from build123d import *

# Parameters (mm, degrees)
SKETCH1_W           = 15.9512
SKETCH1_H           = 13.3096
BOSS_EXTRUDE1_DEPTH = 1.6764
SKETCH2_W           = 2.794
SKETCH2_H           = 1.27
BOSS_EXTRUDE2_DEPTH = 1.016
SKETCH3_R           = 0.9525
CUT_EXTRUDE1_DEPTH  = 2.6764


with BuildPart() as part:
    # Sketch1 → Boss-Extrude1 (new body)
    with BuildSketch(Plane(origin=(0, 0, 0), x_dir=(1, 0, 0), z_dir=(0, 1, 0))):
        with Locations((7.9756, 6.6548)):
            Rectangle(SKETCH1_W, SKETCH1_H)
    extrude(amount=BOSS_EXTRUDE1_DEPTH)

    # Sketch2 → Boss-Extrude2 (add)
    with BuildSketch(Plane(origin=(0, 1.6764, 0), x_dir=(1, 0, 0), z_dir=(0, 1, 0))):
        with Locations((2.413, 6.6548)):
            Rectangle(SKETCH2_W, SKETCH2_H)
        with Locations((6.223, 6.6548)):
            Rectangle(SKETCH2_W, SKETCH2_H)
        with Locations((9.7282, 6.6548)):
            Rectangle(SKETCH2_W, SKETCH2_H)
        with Locations((13.5382, 6.6548)):
            Rectangle(SKETCH2_W, SKETCH2_H)
    extrude(amount=BOSS_EXTRUDE2_DEPTH)

    # Sketch3 → Cut-Extrude1 (cut, through all)
    with BuildSketch(Plane(origin=(0, 1.6764, 0), x_dir=(1, 0, 0), z_dir=(0, 1, 0))):
        with Locations((1.329266667, 12.0396)):
            Circle(SKETCH3_R)
        with Locations((3.987808467, 12.0396)):
            Circle(SKETCH3_R)
        with Locations((6.646350267, 12.0396)):
            Circle(SKETCH3_R)
        with Locations((9.304892067, 12.0396)):
            Circle(SKETCH3_R)
        with Locations((11.963433867, 12.0396)):
            Circle(SKETCH3_R)
        with Locations((14.621975667, 12.0396)):
            Circle(SKETCH3_R)
        with Locations((14.621975667, 1.27)):
            Circle(SKETCH3_R)
        with Locations((11.963433867, 1.27)):
            Circle(SKETCH3_R)
        with Locations((9.304892067, 1.27)):
            Circle(SKETCH3_R)
        with Locations((6.646350267, 1.27)):
            Circle(SKETCH3_R)
        with Locations((3.987808467, 1.27)):
            Circle(SKETCH3_R)
        with Locations((1.329266667, 1.27)):
            Circle(SKETCH3_R)
    extrude(amount=-CUT_EXTRUDE1_DEPTH, mode=Mode.SUBTRACT)


solid = part.part
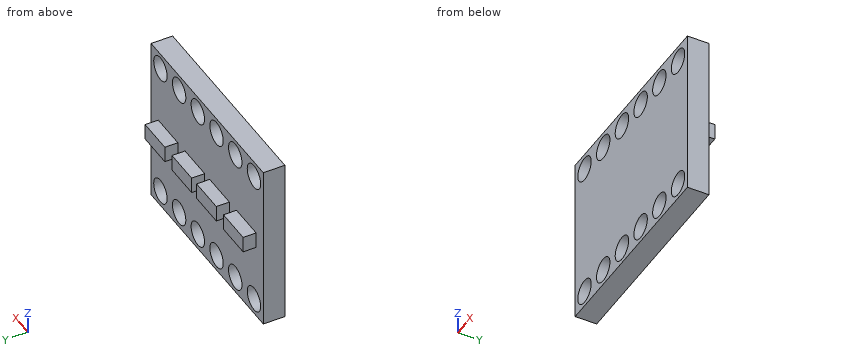
Work out the finished part from the listing and answer in its coordinate system (mm). Give positions to 0.01 mm unless a question says otherwise; leave off trailing zeros. Loops run counter-clockwise (first coordinate to the right, second up) from the corner with the lowest first, then second, coordinate; pieces in that order, holes last. Notation, with made-up numbers: (77.25, 26.25) -> (94.25, 26.25) arc R11 cw to (94.25, 39.25) -> close; hole circle Ø3 at (30, -5). An arc over 180 degrees is marked (long way). Use a Markdown table: item, result. Add a question column.
1) Consider line 1 along Z through (x, y) = (12.5, 1.2); line 2 along Z through (x, y) = (4.25, 1.2); line 3 along Y through (x, z) = (11.75, -4). Determine where each line is inside the solid, lowest interval first.
2) The part is cut by section B-B, the plane z = -1.27. Determine the outline of the cut face in (x, y).
3) The part is cut by section A-A, the plane y = 2.15. Determine the outline of the cut face in (x, z).
4) Each of these flat-tipped pins is pushed along its axis until it touches: P1, Ø3, axis at x = 3.99, z = -1.27, coming from the +Y side; P2, Ø0.8, axis at y = 2.5, z = -6.5, coming from the +X side; P3, Ø0.5, axis at x = 6.5, y = 2, coming from the +Z side. Where does it stop, or does it pass through?
5) The part is cut by section C-C, the plane x = 4. Determine the outline of the cut face in (y, z), plus the area to 3 significant figures.
6) The part is cut by section D-D, the plane y = 0.4. Count the separate pieces of the cut face and the enclosed holes in it, plus the area to 3 significant figures.
Reported:
| question | item | result |
|---|---|---|
| 1 | line 1 | z = -13.31 to -12.83, -11.25 to -2.06, -0.48 to 0 |
| 1 | line 2 | z = -13.31 to -12.96, -11.12 to -2.19, -0.35 to 0 |
| 1 | line 3 | y = 0 to 1.68 |
| 2 | outline | (0, 0) -> (0.38, 0) -> (0.38, 1.68) -> (0, 1.68) -> close; (2.28, 0) -> (3.04, 0) -> (3.04, 1.68) -> (2.28, 1.68) -> close; (4.94, 0) -> (5.69, 0) -> (5.69, 1.68) -> (4.94, 1.68) -> close; (7.6, 0) -> (8.35, 0) -> (8.35, 1.68) -> (7.6, 1.68) -> close; (10.26, 0) -> (11.01, 0) -> (11.01, 1.68) -> (10.26, 1.68) -> close; (12.92, 0) -> (13.67, 0) -> (13.67, 1.68) -> (12.92, 1.68) -> close; (15.57, 0) -> (15.95, 0) -> (15.95, 1.68) -> (15.57, 1.68) -> close |
| 3 | outline | (1.02, -7.29) -> (3.81, -7.29) -> (3.81, -6.02) -> (1.02, -6.02) -> close; (4.83, -7.29) -> (7.62, -7.29) -> (7.62, -6.02) -> (4.83, -6.02) -> close; (8.33, -7.29) -> (11.13, -7.29) -> (11.13, -6.02) -> (8.33, -6.02) -> close; (12.14, -7.29) -> (14.94, -7.29) -> (14.94, -6.02) -> (12.14, -6.02) -> close |
| 4 | P1 | stops at y = 1.68 |
| 4 | P2 | stops at x = 14.94 |
| 4 | P3 | stops at z = -6.02 |
| 5 | outline | (0, -13.31) -> (1.68, -13.31) -> (1.68, -12.99) -> (0, -12.99) -> close; (0, -11.09) -> (1.68, -11.09) -> (1.68, -2.22) -> (0, -2.22) -> close; (0, -0.32) -> (1.68, -0.32) -> (1.68, 0) -> (0, 0) -> close |
| 5 | area | 15.9 mm^2 |
| 6 | separate pieces | 1 |
| 6 | enclosed holes | 12 |
| 6 | area | 178 mm^2 |
